Answer from the drawing. Dimensions are ordinates in mm from the lowest x, y and z of the part. Give positions to 0.01 mm unless a question says otherwise; leave off trailing zeros. Loops run counter-clockwise (first coordinate to the right, second up) from the corner with the lowest first, then second, coordinate; pieces in that order, holes last. Notation, with made-up numbers: M 72.25,56.5 L 117.25,56.5 A13 ccw 117.25,72.5 Z; hole C -13,26.5 d2. An arc over 180 degrees is marked long. Use a Markdown table: item, result.
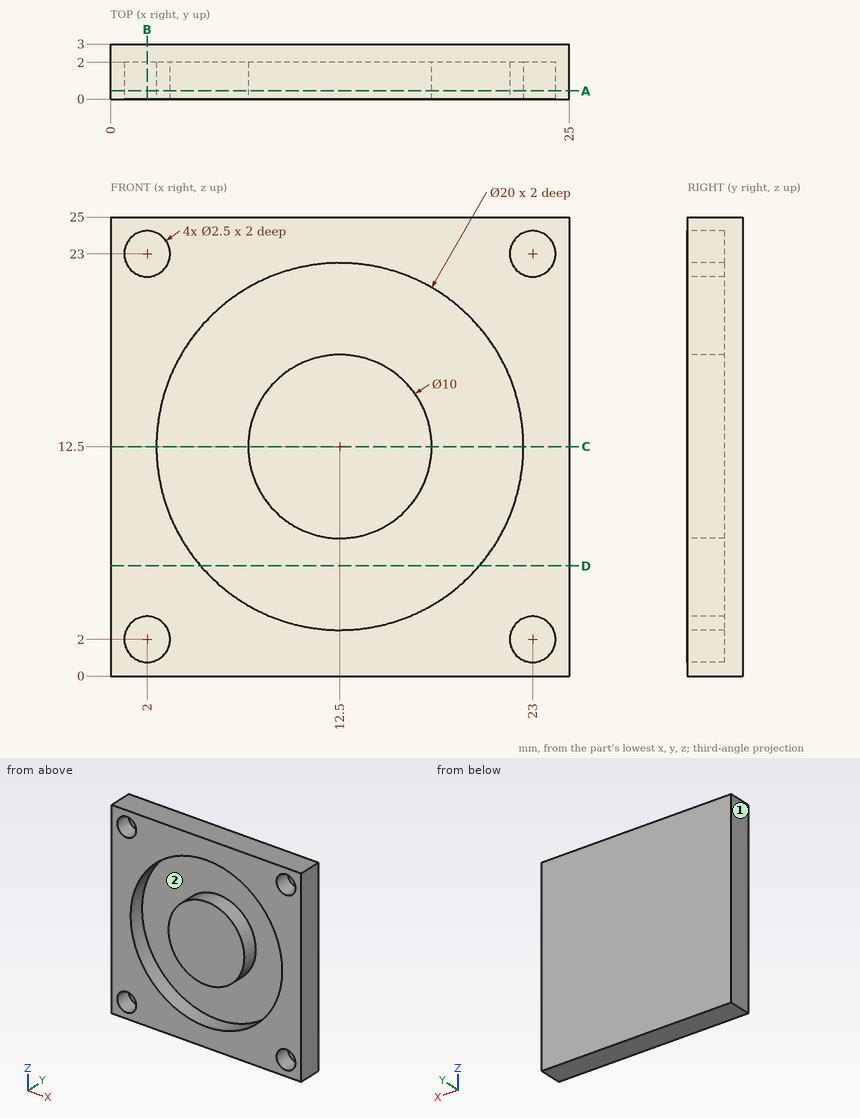
(1) The mould has two halves that part along Z. Classify the marked faces 1 and 2: released by +Z, released by -Z, zero draft, split by the parting line, or undercut.
Entries:
| item | result |
|---|---|
| face 1 | zero draft |
| face 2 | undercut |
(2) A cutting plane is placed at C-C (z = 12.5). Write down the section's boundary in (x, y).
Entries:
| item | result |
|---|---|
| outline | M 0,0 L 2.5,0 L 2.5,2 L 7.5,2 L 7.5,0 L 17.5,0 L 17.5,2 L 22.5,2 L 22.5,0 L 25,0 L 25,3 L 0,3 Z |
(3) Consider probe 1 along Z at (x, y) = (2, 1.2); probe 2 along Z at (x, y) = (12.5, 1.1); probe 3 along X at (y, z) = (1.1, 1.25). Determine where each line is inside the solid, lowest interval first. Write a range as [from, to].
Entries:
| item | result |
|---|---|
| probe 1 | z = [0, 0.75], [3.25, 21.75], [24.25, 25] |
| probe 2 | z = [0, 2.5], [7.5, 17.5], [22.5, 25] |
| probe 3 | x = [0, 1], [3, 22], [24, 25] |
(4) A cutting plane is placed at D-D (z = 6). Write down the section's boundary in (x, y).
Entries:
| item | result |
|---|---|
| outline | M 0,0 L 4.9,0 L 4.9,2 L 20.1,2 L 20.1,0 L 25,0 L 25,3 L 0,3 Z |
(5) A cutting plane is placed at B-B (x = 2). Write down the section's boundary in (y, z), and give its area (3 significant figures).
Entries:
| item | result |
|---|---|
| outline | M 0,0 L 3,0 L 3,25 L 0,25 L 0,24.25 L 2,24.25 L 2,21.75 L 0,21.75 L 0,3.25 L 2,3.25 L 2,0.75 L 0,0.75 Z |
| area | 65.0 mm² |
(6) Given P1, Ø10, axis at x = 8.5, z = 17.5, coming from the -Y side; P2, Ø1.5, axis at x = 23, z = 23, coming from the -Y side, each flat-ended and moving along its own axis, determine where each tip first touches the part or whether it passes through.
Entries:
| item | result |
|---|---|
| P1 | stops at y = 0 |
| P2 | stops at y = 2 |
(7) A cutting plane is placed at A-A (y = 0.45). Write down the section's boundary in (x, z).
Entries:
| item | result |
|---|---|
| outline | M 0,0 L 25,0 L 25,25 L 0,25 Z; C 12.5,12.5 d10; hole C 2,2 d2.5; hole C 2,23 d2.5; hole C 12.5,12.5 d20; hole C 23,2 d2.5; hole C 23,23 d2.5 |
